Autodesk Inventor part; units mm, degrees
ref_plane "YZ Plane" through (0, 0, 0) normal (1, 0, 0) x (0, 1, 0)
ref_plane "XZ Plane" through (0, 0, 0) normal (0, 1, 0) x (-1, 0, 0)
ref_plane "XY Plane" through (0, 0, 0) normal (0, 0, 1) x (1, 0, 0)
sketch "Эскиз1" plane through (0, 0, 0) normal (0, 0, 1) x (1, 0, 0)
  line L0 (0, 0) -> (20, 0)
  line L1 (20, 0) -> (20, 30)
  line L2 (20, 30) -> (0, 30)
  line L3 (0, 30) -> (0, 0)
  dimension "d0" = 20
  dimension "d1" = 30
revolve "Вращение1" add sketch "Эскиз1" angle 360 about axis through (0, 0, 0) along (1, 0, 0)
sketch "Эскиз2" plane through (0, 0, 0) normal (-1, 0, 0) x (0, 0, 1)
  circle A0 centre (0, 0) radius 30 construction
  circle A1 centre (0, 0) radius 30
  line L0 (-3, 29.8496) -> (-3, 26.8496)
  line L1 (3, 29.8496) -> (3, 26.8496)
  arc A2 (-3, 26.8496) -> (3, 26.8496) centre (0, 26.8496) ccw
  line L2 (-29.8496, -3) -> (-26.8496, -3)
  line L3 (-29.8496, 3) -> (-26.8496, 3)
  arc A3 (-26.8496, -3) -> (-26.8496, 3) centre (-26.8496, 0) ccw
  line L4 (3, -29.8496) -> (3, -26.8496)
  line L5 (-3, -29.8496) -> (-3, -26.8496)
  arc A4 (3, -26.8496) -> (-3, -26.8496) centre (0, -26.8496) ccw
  line L6 (29.8496, 3) -> (26.8496, 3)
  line L7 (29.8496, -3) -> (26.8496, -3)
  arc A5 (26.8496, 3) -> (26.8496, -3) centre (26.8496, 0) ccw
  dimension "d3" = 3
  dimension "d4" = 3
  dimension "d5" = 3
  dimension "d8" = 360
extrude "Выдавливание1" cut sketch "Эскиз2" against normal blind 20 contours A1 L7 A5 L6 | L1 A2 L0 A1 | A1 L5 A4 L4 | L3 A3 L2 A1
sketch "Эскиз3" plane through (0, 0, 26.8496) normal (-1, 0, 0) x (0, 0, 1)
  line L0 (-26.8496, 0) -> (-21.8496, 0) construction
  dimension "d12" = 5
hole "Отверстие1" at (0, 0, 5) direction (1, 0, 0) diameter 14 depth 8 tip angle 118 countersink diameter 19 countersink angle 90
properties part number "711114"
Here's how the part is built. I have some questions about the finished solid (model axes, mm). A direction names the side the tool comes from. Give positions to 0.01 mm unless a question says otherwise; leave off trailing zeros. Order: outer loops, then holes, each group sorted by start corner. A loop starts at its lowest first (then second) coordinate and runs counter-clockwise, first axis right, second up. Notation, with made-up numbers: (8, -8.5) -> (35, -8.5) arc R27 cw to (35, 15.5) -> close; hole circle Ø6 at (-8, -6.75). An arc over 180 degrees is marked (long way). Use a Markdown table: item, result. Add a question column.
Item 1: Imagine slicing it at D-D on y = -11. Please give me the cut outline in (x, z).
Item 2: Imagine slicing it at C-C on x = 13.5. Please give me the cut outline in (y, z), plus the area to 3 significant figures.
Item 3: For faces 1 (the face through (10, -3, 28)), 2 (the face through (5, 0, -2)), 3 (the face through (10, -28, -3)), which set-ups out of +Z, -Z, +X, -X, +Y, -Y let a thin tool reach every point of the face, with its end or its side?
Item 4: Imagine slicing it at A-A on x = 5. Please give me the cut outline in (y, z).
Item 5: I need wall thicknesses on line 1 (Z direction, x = 6.75, y = 0); line 2 (Y direction, x = 5.4, z = 5); line 3 (Y direction, x = 6.75, z = 7.5). Which ranges of each line are inside material? Lowest first, please.
Item 6: Will these pins go through, and if not, where does the flat tip stop? pin 1 (3.5 mm diameter, centred on x = 14.5, y = -29, fed in from -Z); pin 2 (1.5 mm diameter, centred on x = 10, z = -28.5, fed in from -Y); pin 3 (8 mm diameter, centred on x = 7.5, y = -4.5, fed in from +Z).
Item 7: Imagine slicing it at B-B on z = 25.5. Please give me the cut outline in (x, y), plus the area to 3 significant figures.
Item 8: If we mould it in two halves opening along Y, with no side actions, what happens to faces 4 (the face through (9.86, 21.416, -21.009)), 5 (the face through (0, 0, -6)), 6 (the face through (10, 3, 28))? For each: pulls with the +Y half, pulls with the -Y half, needs draft (parallel to the pull), parting line crosses it, or undercut.
Data:
| question | item | result |
|---|---|---|
| 1 | outline | (0, -27.91) -> (20, -27.91) -> (20, 27.91) -> (0, 27.91) -> close |
| 2 | outline | (-29.85, -3) arc R30 ccw to (-3, -29.85) -> (-3, -26.85) arc R3 cw to (3, -26.85) -> (3, -29.85) arc R30 ccw to (29.85, -3) -> (26.85, -3) arc R3 cw to (26.85, 3) -> (29.85, 3) arc R30 ccw to (3, 29.85) -> (3, 26.85) arc R3 cw to (-3, 26.85) -> (-3, 29.85) arc R30 ccw to (-29.85, 3) -> (-26.85, 3) arc R3 cw to (-26.85, -3) -> close |
| 2 | area | 2,700 mm² |
| 3 | face 1 | +Z, +X, -X |
| 3 | face 2 | -X |
| 3 | face 3 | +X, -X, -Y |
| 4 | outline | (-29.85, -3) arc R30 ccw to (-3, -29.85) -> (-3, -26.85) arc R3 cw to (3, -26.85) -> (3, -29.85) arc R30 ccw to (29.85, -3) -> (26.85, -3) arc R3 cw to (26.85, 3) -> (29.85, 3) arc R30 ccw to (3, 29.85) -> (3, 26.85) arc R3 cw to (-3, 26.85) -> (-3, 29.85) arc R30 ccw to (-29.85, 3) -> (-26.85, 3) arc R3 cw to (-26.85, -3) -> close; hole circle Ø14 at (0, 5) |
| 5 | line 1 | z = -23.85 to -2, 12 to 23.85 |
| 5 | line 2 | y = -29.58 to -7, 7 to 29.58 |
| 5 | line 3 | y = -29.05 to -6.54, 6.54 to 29.05 |
| 6 | pin 1 | stops at z = -12.55 |
| 6 | pin 2 | stops at y = -11.4 |
| 6 | pin 3 | stops at z = 29.85 |
| 7 | outline | (0, -15.8) -> (20, -15.8) -> (20, -2.68) -> (0, -2.68) -> close; (0, 2.68) -> (20, 2.68) -> (20, 15.8) -> (0, 15.8) -> close |
| 7 | area | 525 mm² |
| 8 | face 4 | pulls with the +Y half |
| 8 | face 5 | needs draft |
| 8 | face 6 | undercut |
